Job drawing, mm, ordinate dimensions from the low corner. One solid piece. A direction names the side the tool comes from. Round coordinates to 2 decimals unless told otherwise and drop trailing zeros. Loops run counter-clockwise (first coordinate to the right, second up) from the corner with the lowest first, then second, coordinate; pieces in that order, holes last.
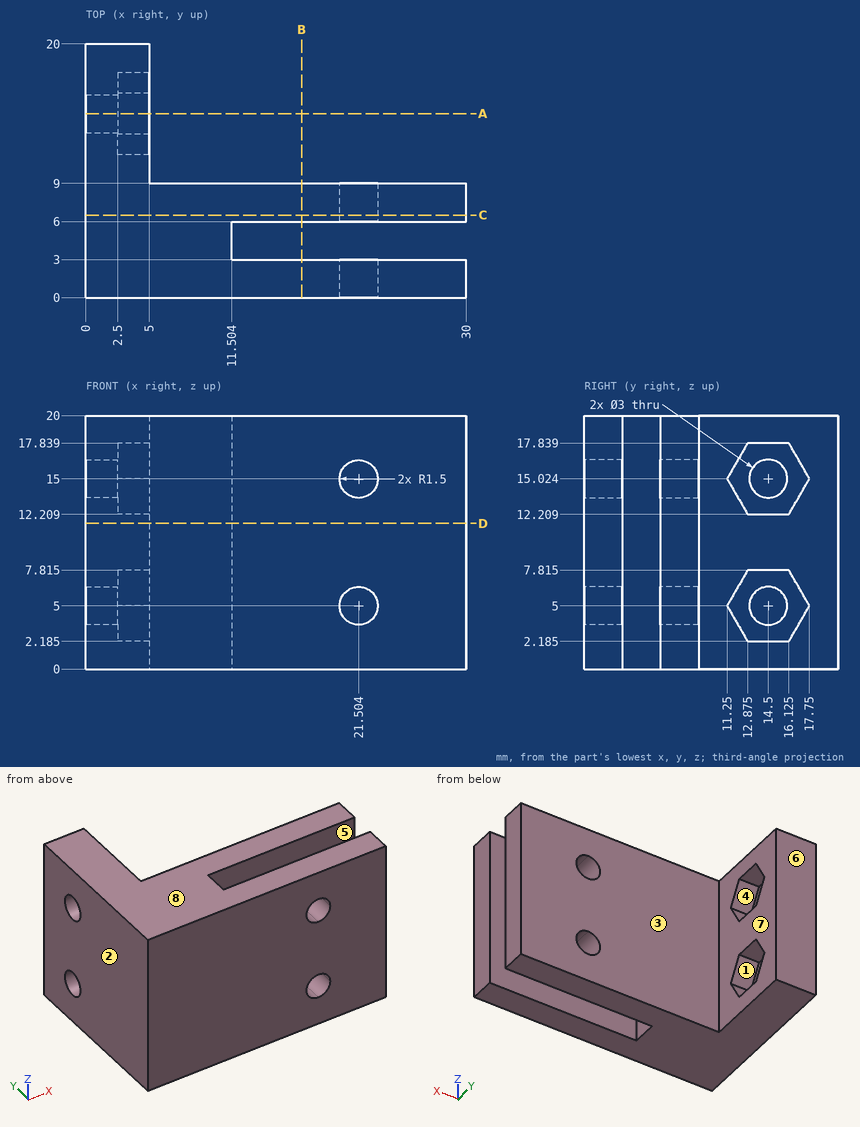
1) Slice it at D-D, the plane z = 11.5. Give the cut face in (x, y).
Values:
outline: (0, 0) - (30, 0) - (30, 3) - (11.5, 3) - (11.5, 6) - (30, 6) - (30, 9) - (5, 9) - (5, 20) - (0, 20) - close
2) Slice it at C-C, the plane y = 6.5. Give the cut face in (x, z).
Values:
outline: (0, 0) - (30, 0) - (30, 20) - (0, 20) - close; hole circle Ø3 at (21.5, 5); hole circle Ø3 at (21.5, 15)
3) Slice it at A-A, the plane y = 14.5. Give the cut face in (x, z) (1 decimal).
Values:
outline: (0, 0) - (5, 0) - (5, 2.2) - (2.5, 2.2) - (2.5, 3.5) - (0, 3.5) - close; (0, 6.5) - (2.5, 6.5) - (2.5, 7.8) - (5, 7.8) - (5, 12.2) - (2.5, 12.2) - (2.5, 13.5) - (0, 13.5) - close; (0, 16.5) - (2.5, 16.5) - (2.5, 17.8) - (5, 17.8) - (5, 20) - (0, 20) - close
4) Tool access for the marked faces 4, 5, 6, 7 and 8: list every direction of +Z, -Z, +X, -X, +Y, -Y with a clear straight run to the whole face (end or side of a thin tool).
Values:
face 4: +X
face 5: +Z, -Z, +X
face 6: +Z, -Z, +X, -X, +Y
face 7: +Z, -Z, +X, +Y
face 8: +Z, +X, -X, +Y, -Y
5) Mould opens along Y. For the marked faces 1, 2 and 3 say: released by +Y, released by -Y, zero draft, split by the parting line, or undercut.
Values:
face 1: undercut
face 2: zero draft
face 3: released by +Y
6) Slice it at B-B, the plane x = 17. Give the cut face in (y, z), then the cut area to 3 significant figures.
Values:
outline: (0, 0) - (3, 0) - (3, 20) - (0, 20) - close; (6, 0) - (9, 0) - (9, 20) - (6, 20) - close
area: 120 mm2
7) Drop flat-ended pins along their axis: pin 1 Ø8 at (x, z) = (16.5, 11) entering from +Y; pin 2 Ø1.5 at (y, z) = (4, 9) entering from +X; pin 3 Ø5.5 at (y, z) = (15, 10.5) entering from +X; pin 4 Ø1.8 at (y, z) = (14.5, 5) entering from -X. Give the stop position or say it passes through.
Values:
pin 1: stops at y = 9
pin 2: stops at x = 11.5
pin 3: stops at x = 5
pin 4: passes through
8) Wall check: line 1 along Y through (x, z) = (21, 2.5); line 2 along Y through (x, z) = (2.05, 5); line 3 along X through (y, z) = (18.75, 17). Give the ranges that are in metal, low to high.
Values:
line 1: y = 0 to 3, 6 to 9
line 2: y = 0 to 13, 16 to 20
line 3: x = 0 to 5
